Source: CAD feature listing. Evaluate the final solid. Frame: model axes, mm. Give positions to 0.01 mm unless a question says otherwise; leave off trailing zeros. Write each loop counter-clockwise with the first axis right and the second up, starting at its lowest first coordinate (ties: lowest second). Pieces come first, ordered by that corner, then holes. Notation, with made-up numbers: (41.5, -3.75) - (90.5, -3.75) arc R33 cw to (90.5, 32.25) - close; hole circle Ø10 at (-29.5, -2). An arc over 180 degrees is marked (long way). Answer as a JSON object with one key per item and string values. Group by question number.
from build123d import *

# Parameters (mm, degrees)
SKETCH1_R           = 10
SKETCH1_R_2         = 1.55
SKETCH1_R_3         = 12.525
SKETCH1_R_4         = 2.25
SKETCH1_R_5         = 2
SKETCH1_W           = 8
SKETCH1_H           = 5
BOSS_EXTRUDE1_DEPTH = 1.5


with BuildPart() as part:
    # Sketch1 → Boss-Extrude1 (new body)
    with BuildSketch(Plane(origin=(0, 0, 0), x_dir=(1, 0, 0), z_dir=(0, 1, 0))):
        with BuildLine():
            Line((44.790320824, 89.722222222), (71.664513318, 35.555555556))
            ThreePointArc((71.664513318, 35.555555556), (0, -80), (-71.664513318, 35.555555556))
            Line((-71.664513318, 35.555555556), (-44.790320824, 89.722222222))
            ThreePointArc((-44.790320824, 89.722222222), (0, 117.5), (44.790320824, 89.722222222))
        make_face()
        Circle(SKETCH1_R, mode=Mode.SUBTRACT)
        with Locations((-12.990381057, -7.5)):
            Circle(SKETCH1_R_2, mode=Mode.SUBTRACT)
        with Locations((12.990381057, -7.5)):
            Circle(SKETCH1_R_2, mode=Mode.SUBTRACT)
        with Locations((0, 15)):
            Circle(SKETCH1_R_2, mode=Mode.SUBTRACT)
        with Locations((0, 67.5)):
            Circle(SKETCH1_R_3, mode=Mode.SUBTRACT)
        with Locations((40, 67.5)):
            Circle(SKETCH1_R_4, mode=Mode.SUBTRACT)
        with Locations((70, 0)):
            Circle(SKETCH1_R_4, mode=Mode.SUBTRACT)
        with Locations((56.631189606, -41.14496766)):
            Circle(SKETCH1_R_4, mode=Mode.SUBTRACT)
        with Locations((21.631189606, -66.573956141)):
            Circle(SKETCH1_R_4, mode=Mode.SUBTRACT)
        with Locations((-21.631189606, -66.573956141)):
            Circle(SKETCH1_R_4, mode=Mode.SUBTRACT)
        with Locations((-56.631189606, -41.14496766)):
            Circle(SKETCH1_R_4, mode=Mode.SUBTRACT)
        with Locations((-70, 0)):
            Circle(SKETCH1_R_4, mode=Mode.SUBTRACT)
        with Locations((28.284271247, 95.784271247)):
            Circle(SKETCH1_R_4, mode=Mode.SUBTRACT)
        with Locations((0, 107.5)):
            Circle(SKETCH1_R_4, mode=Mode.SUBTRACT)
        with Locations((-28.284271247, 95.784271247)):
            Circle(SKETCH1_R_4, mode=Mode.SUBTRACT)
        with Locations((-40, 67.5)):
            Circle(SKETCH1_R_4, mode=Mode.SUBTRACT)
        with Locations((-50.153461651, 44.654711284)):
            Circle(SKETCH1_R_4, mode=Mode.SUBTRACT)
        with Locations((-60.306923303, 21.809422569)):
            Circle(SKETCH1_R_4, mode=Mode.SUBTRACT)
        with Locations((50.153461651, 44.654711284)):
            Circle(SKETCH1_R_4, mode=Mode.SUBTRACT)
        with Locations((60.306923303, 21.809422569)):
            Circle(SKETCH1_R_4, mode=Mode.SUBTRACT)
        with Locations((0, 87.707259422)):
            Circle(SKETCH1_R_2, mode=Mode.SUBTRACT)
        with Locations((-17.5, 57.396370289)):
            Circle(SKETCH1_R_2, mode=Mode.SUBTRACT)
        with Locations((17.5, 57.396370289)):
            Circle(SKETCH1_R_2, mode=Mode.SUBTRACT)
        with Locations((-23.249483938, 93.662215055)):
            Circle(SKETCH1_R_5, mode=Mode.SUBTRACT)
        with Locations((17.859623375, 37.399603775)):
            Circle(SKETCH1_R_5, mode=Mode.SUBTRACT)
        with Locations((0, 47.5)):
            Rectangle(SKETCH1_W, SKETCH1_H, mode=Mode.SUBTRACT)
        with Locations((-1.994503305, -58.420364393)):
            Rectangle(SKETCH1_W, SKETCH1_H, mode=Mode.SUBTRACT)
        with Locations((-34.37581539, 50)):
            Rectangle(SKETCH1_W, SKETCH1_H, mode=Mode.SUBTRACT)
        with Locations((34.136464886, 49.290075758)):
            Rectangle(SKETCH1_W, SKETCH1_H, mode=Mode.SUBTRACT)
        with Locations((54.012994775, -0.420504721)):
            Rectangle(SKETCH1_W, SKETCH1_H, mode=Mode.SUBTRACT)
        with Locations((-56.673760324, -13.260168312)):
            Rectangle(SKETCH1_W, SKETCH1_H, mode=Mode.SUBTRACT)
        with Locations((-0.046638908, 98.711772009)):
            Rectangle(SKETCH1_W, SKETCH1_H, mode=Mode.SUBTRACT)
    extrude(amount=BOSS_EXTRUDE1_DEPTH)


solid = part.part
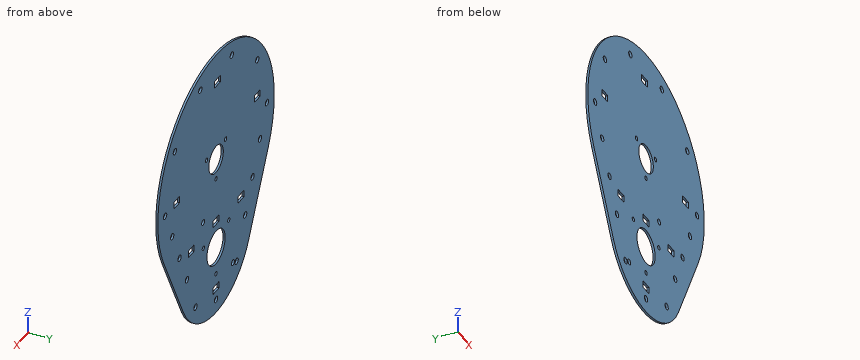
Q1. First-contact query: pin 1 Ø2.5 at (x, z) = (0, -15) entering from -Y. Flat tip, straight axial feed; report the tip coordinate or a pass-through.
Q2. Section B-B on z = 0. Return the cut outline in (x, y).
Q3. Ray query, probe 1 along X at (y, z) = (1, 7.5); probe 2 along Z at (x, y) = (3, 0.3); probe 3 along Z at (x, y) = (-7.5, 0.2). Return the intervals inside material, ascending. Write a range as [from, to].
Q4. Section A-A on z = -107.5. Return the cut outline in (x, y).
Q5. Section C-C on y = 0.9. State how many separate pieces and enclosed holes the cut face has, then the cut area to 3 significant figures.
Q6. Section D-D on z = 28.5. Return the cut outline in (x, y).
Taken from the geometry:
{
 "1": {"pin 1": "passes through"},
 "2": {"outline": "(-80, 0) - (-72.25, 0) - (-72.25, 1.5) - (-80, 1.5) - close; (-67.75, 0) - (-10, 0) - (-10, 1.5) - (-67.75, 1.5) - close; (10, 0) - (50.01, 0) - (50.01, 1.5) - (10, 1.5) - close; (58.01, 0) - (67.75, 0) - (67.75, 1.5) - (58.01, 1.5) - close; (72.25, 0) - (80, 0) - (80, 1.5) - (72.25, 1.5) - close"},
 "3": {"probe 1": "x = [-79.65, -14.54], [-11.44, -6.61], [6.61, 11.44], [14.54, 79.65]", "probe 2": "z = [-117.41, -101.21], [-96.21, -79.66], [-55.34, -50], [-45, -9.54], [9.54, 79.94]", "probe 3": "z = [-116.93, -77.53], [-57.47, -6.61], [6.61, 79.65]"},
 "4": {"outline": "(-30, 0) - (-2.25, 0) - (-2.25, 1.5) - (-30, 1.5) - close; (2.25, 0) - (30, 0) - (30, 1.5) - (2.25, 1.5) - close"},
 "5": {"separate pieces": "1", "enclosed holes": "32", "area": "22,200 mm²"},
 "6": {"outline": "(-74.75, 0) - (74.75, 0) - (74.75, 1.5) - (-74.75, 1.5) - close"}
}
